Geometry: final body of the model. Coordinates: model frame, mm. A direction names the side the tool comes from. Give positions to 0.01 mm unless a question says otherwise; leave off trailing zeros.
from build123d import *

# Parameters (mm, degrees)
SKETCH1_W           = 150
SKETCH1_H           = 150
SKETCH1_R           = 1.65
SKETCH1_W_2         = 5
SKETCH1_H_2         = 15
BOSS_EXTRUDE1_DEPTH = 8


with BuildPart() as part:
    # Sketch1 → Boss-Extrude1 (new body)
    with BuildSketch(Plane(origin=(0, 0, 0), x_dir=(1, 0, 0), z_dir=(0, 1, 0))):
        with Locations((75, 75)):
            Rectangle(SKETCH1_W, SKETCH1_H)
        with Locations((102.5, 75)):
            Circle(SKETCH1_R, mode=Mode.SUBTRACT)
        with Locations((47.5, 75)):
            Circle(SKETCH1_R, mode=Mode.SUBTRACT)
        with Locations((102.5, 52.5)):
            Rectangle(SKETCH1_W_2, SKETCH1_H_2, mode=Mode.SUBTRACT)
        with Locations((102.5, 97.5)):
            Rectangle(SKETCH1_W_2, SKETCH1_H_2, mode=Mode.SUBTRACT)
        with Locations((47.5, 52.5)):
            Rectangle(SKETCH1_W_2, SKETCH1_H_2, mode=Mode.SUBTRACT)
        with Locations((47.5, 97.5)):
            Rectangle(SKETCH1_W_2, SKETCH1_H_2, mode=Mode.SUBTRACT)
    extrude(amount=BOSS_EXTRUDE1_DEPTH)


solid = part.part
Q1. Ray query, line 1 along X through (y, z) = (5, -75); line 2 along Z through (x, y) = (47.5, 5); line 3 along X through (y, z) = (7.5, -47). Return the intervals inside material, ascending.
Filled sheet:
line 1: x = 0 to 45.85, 49.15 to 100.85, 104.15 to 150
line 2: z = -150 to -105, -90 to -76.65, -73.35 to -60, -45 to 0
line 3: x = 0 to 45, 50 to 100, 105 to 150
Q2. Access query for faces 1 (the flat face through (100, 4, -52)), 2 (the flat face through (74, 4, -150)). Directions: +Z, -Z, +X, -X, +Y, -Y. A direction counts if a zero-diameter tool reaches every point of the face in a straight line with its end or side. Return the directions, or none.
Filled sheet:
face 1: +Y, -Y
face 2: -Z, +X, -X, +Y, -Y
Q3. Pull-direction query (Z, two-part tool) for faces 3 (the flat face through (0, 4, -74)), 4 (the flat face through (100, 4, -97)), 5 (the flat face through (74, 4, 0)); classes: released by +Z, released by -Z, zero draft, split by the parting line, or undercut.
Filled sheet:
face 3: zero draft
face 4: undercut
face 5: released by +Z
